Geometry: final body of the model. Coordinates: model frame, mm. Face numbers are marked on the shaded views. A direction names the side the tool comes from. Give positions to 0.01 mm unless a question says otherwise; leave off trailing zeros. Loops run counter-clockwise (first coordinate to the right, second up) from the corner with the lowest first, then second, coordinate; pieces in that order, holes last. Notation, with made-up numbers: M -35,-15 L 7,-15 A22 ccw 7,18 Z; hole C 70.5,-7 d2. An arc over 180 degrees is marked long. One line per question, with ' | ' between items. Start each with the question number.
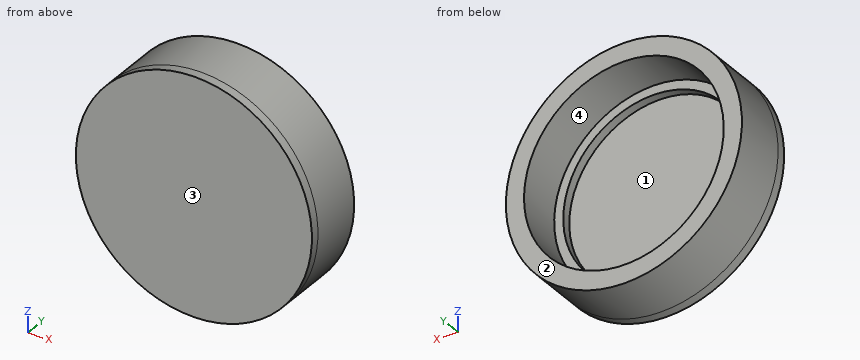
from build123d import *

# Parameters (mm, degrees)
ESQUISSE1_R        = 13
ESQUISSE1_R_2      = 11
BOSS_EXTRU_1_DEPTH = 6
BOSS_EXTRU_2_START = 1
ESQUISSE2_R        = 13
BOSS_EXTRU_2_DEPTH = 1
ESQUISSE3_R        = 11
ESQUISSE3_R_2      = 10
BOSS_EXTRU_3_DEPTH = 1


with BuildPart() as part:
    # Esquisse1 → Boss.-Extru.1 (new body)
    with BuildSketch(Plane(origin=(0, 0, 0), x_dir=(1, 0, 0), z_dir=(0, 1, 0))):
        with Locations(Location((0, 0, 0), (0, 0, 270))):
            Circle(ESQUISSE1_R)
        with Locations(Location((0, 0, 0), (0, 0, 270))):
            Circle(ESQUISSE1_R_2, mode=Mode.SUBTRACT)
    extrude(amount=BOSS_EXTRU_1_DEPTH)

    # Esquisse2 → Boss.-Extru.2 (add)
    with BuildSketch(Plane.XZ.offset(BOSS_EXTRU_2_START)):
        with Locations(Location((0, 0, 0), (0, 0, 270))):
            Circle(ESQUISSE2_R)
    extrude(amount=-BOSS_EXTRU_2_DEPTH)

    # Esquisse3 → Boss.-Extru.3 (add)
    with BuildSketch(Plane(origin=(0, 0, 0), x_dir=(1, 0, 0), z_dir=(0, 1, 0))):
        with Locations(Location((0, 0, 0), (0, 0, 270))):
            Circle(ESQUISSE3_R)
        with Locations(Location((0, 0, 0), (0, 0, 270))):
            Circle(ESQUISSE3_R_2, mode=Mode.SUBTRACT)
    extrude(amount=BOSS_EXTRU_3_DEPTH)


solid = part.part
Q1. Section C-C, the plane z = 0. Output: boundary loops of the cut face in (x, y).
Q2. Contact query for flat-ended pins moving along their axis: pin 1 (4 mm diameter, centred on y = 0.5, z = 7.5, fed in from -X); pin 2 (2 mm diameter, centred on x = 1, z = 9.5, fed in from +Y); pin 3 (1.5 mm diameter, centred on x = 6, y = 1, fed in from +Z). Output: stop coordinate, or through.
Q3. Draft query along Z for the marked faces 1 and 2. Return one class per face: released by +Z, released by -Z, zero draft, split by the parting line, or undercut.
Q4. Set-up query: the marked faces 3 and 4. Return all of +Z, -Z, +X, -X, +Y, -Y with unobstructed straight access to the full face (end or side cutting, diameter ignored); none if empty.
Q5. Section A-A, the plane x = 0. Output: boundary loops of the cut face in (y, z).
Q6. Material intervals for L1, parallel to X at y = 0.55, z = 0; L2, parallel to X at y = 3.9, z = 0; L3, parallel to Y at x = 7.75, z = 7.25, sorted ascending.
Q7. Section B-B, the plane y = 1.75. Output: boundary loops of the cut face in (x, z).
Model answer:
1) outline: M -13,-1 L 13,-1 L 13,6 L 11,6 L 11,1 L 10,1 L 10,0 L -10,0 L -10,1 L -11,1 L -11,6 L -13,6 Z
2) pin 1: stops at x = -11.78 | pin 2: stops at y = 1 | pin 3: stops at z = 11.89
3) face 1: undercut | face 2: zero draft
4) face 3: +Z, -Z, +X, -X, -Y | face 4: +Y
5) outline: M -1,-13 L 6,-13 L 6,-11 L 1,-11 L 1,-10 L 0,-10 L 0,10 L 1,10 L 1,11 L 6,11 L 6,13 L -1,13 Z
6) L1: x = -13 to -10, 10 to 13 | L2: x = -13 to -11, 11 to 13 | L3: y = -1 to 1
7) outline: C 0,0 d26; hole C 0,0 d22
